Input: part model. Units: mm. Frame: model coordinates. A direction names the side the tool comes from. Round coordinates to 2 decimals unless told otherwise and drop trailing zeros. Loops run counter-clockwise (first coordinate to the right, second up) from the corner with the lowest first, then second, coordinate; pieces in that order, holes last. Notation, with made-up numbers: (-36.75, 69.5) -> (-1.75, 69.5) arc R22 cw to (-1.75, 94.5) -> close; hole circle Ø3 at (78, 26). An arc over 180 degrees is marked (long way). Answer in a Markdown table with one row per item. Add a question column.
Q1. Section A-A, the plane y = -0.5. Output: boundary loops of the cut face in (x, z).
Q2. Mould query, pull axis Z, two halves, no side actions, for faces 1 (the face through (-4.757, 11.598, -0.528)), 2 (the face through (-0.54, -2.44, -0.49)), 3 (the face through (-2, -2, 0)). Classes: pulls with the +Z half, pulls with the -Z half, needs draft (parallel to the pull), parting line crosses it, or undercut.
Q3. Ray query, L1, parallel to Y at x = 8, z = -0.6; L2, parallel to Y at x = 3.75, z = -0.3; L3, parallel to X at y = -6.75, z = -0.1. Return the intervals inside material, ascending. Write a range as from..to.
Q4. Reachability of faces 4 (the face through (4.94, 12.67, -0.49)), 5 (the face through (5.637, 2.848, -0.493)), 6 (the face through (7.3, 0, -0.5)), 7 (the face through (-7.3, 0, -0.5)) from +Z, -Z, +X, -X, +Y, -Y: full face, straight path, thin tool, end or side. Return the list, or none.
Q5. Section B-B, the plane x = -7.75. Give the number of separate pieces and of enclosed holes in the cut face, and give its area (3 significant figures).
Q6. Pin query (flat end, axial travel): pin 1 (0.5 mm diameter, centred on x = 2.5, z = -0.5, fed in from +Y); pin 2 (0.5 mm diameter, centred on y = -7.5, z = -0.5, fed in from -X). Return the tip coordinate at first contact, or that it passes through.
```python
from build123d import *

# Parameters (mm, degrees)
SKETCH1_R           = 2.5
BOSS_EXTRUDE1_DEPTH = 1
BOSS_EXTRUDE2_DEPTH = 1
CUT_EXTRUDE1_START  = -1
SKETCH5_R           = 0.5
CUT_EXTRUDE1_DEPTH  = 20.707970143
CIRPATTERN4_COUNT   = 8


with BuildPart() as part:
    # Sketch1 → Boss-Extrude1 (new body)
    with BuildSketch(Plane.XY):
        Polygon((-6, 0), (-6, 4.000001453), (-8.5, 4.000001453), (-8.5, 6), (-6, 6), (-4.242640687, 4.242640687), (-1.414212535, 7.071068839), (-3.181979488, 8.838835792), (-1.767766953, 10.253048327), (0, 8.485281374), (0, 6), (4.000001453, 6), (4.000001453, 8.5), (6, 8.5), (6, 6), (4.242640687, 4.242640687), (7.071068839, 1.414212535), (8.838835792, 3.181979488), (10.253048327, 1.767766953), (8.485281374, 0), (6, 0), (6, -4.000001453), (8.5, -4.000001453), (8.5, -6), (6, -6), (4.242640687, -4.242640687), (1.414212535, -7.071068839), (3.181979488, -8.838835792), (1.767766953, -10.253048327), (0, -8.485281374), (0, -6), (-4.000001453, -6), (-4.000001453, -8.5), (-6, -8.5), (-6, -6), (-4.242640687, -4.242640687), (-7.071068839, -1.414212535), (-8.838835792, -3.181979488), (-10.253048327, -1.767766953), (-8.485281374, 0), align=None)
        Circle(SKETCH1_R, mode=Mode.SUBTRACT)
    extrude(amount=-BOSS_EXTRUDE1_DEPTH)

    # Sketch2 → Boss-Extrude2 (add)
    with BuildSketch(Plane.XY):
        with BuildLine():
            Line((6, 8.5), (4.000001453, 8.5))
            add(Edge.make_bspline(
                [(4.000001453, 8.5), (4.535044761, 9.851871254), (2.785677296, 10.626331859), (1.69748686, 10.584769031)],
                knots=[0, 0, 0, 0, 1, 1, 1, 1], degree=3))
            ThreePointArc((1.69748686, 10.584769031), (5.000000726, 12.6701636), (8.302514593, 10.584769031))
            add(Edge.make_bspline(
                [(6, 8.5), (5.464956692, 9.851871254), (7.214324157, 10.626331859), (8.302514593, 10.584769031)],
                knots=[0, 0, 0, 0, 1, 1, 1, 1], degree=3))
        make_face()
    boss_extrude2 = extrude(amount=-BOSS_EXTRUDE2_DEPTH)

    # Sketch5 → Cut-Extrude1 (cut)
    with BuildSketch(Plane(origin=(-8.102008287, 0, -8.102008287), x_dir=(0, -1, 0), z_dir=(0.707106781, 0, 0.707106781)).offset(CUT_EXTRUDE1_START)):
        with Locations((-11.065369039, 3.772340366)):
            Circle(SKETCH5_R)
    cut_extrude1 = extrude(amount=CUT_EXTRUDE1_DEPTH, mode=Mode.SUBTRACT)

    # CirPattern4: Boss-Extrude2, Cut-Extrude1 ×8 about axis
    cirpattern4_axis = Axis((0, 0, 0), (0, 0, 1))
    for i in range(1, CIRPATTERN4_COUNT):
        add(boss_extrude2.rotate(cirpattern4_axis, i * 360 / CIRPATTERN4_COUNT))
        add(cut_extrude1.rotate(cirpattern4_axis, i * 360 / CIRPATTERN4_COUNT), mode=Mode.SUBTRACT)


solid = part.part
```
Answer block:
| question | item | result |
|---|---|---|
| 1 | outline | (-8.99, -1) -> (-2.45, -1) -> (-2.45, 0) -> (-8.99, 0) -> close; (2.45, -1) -> (6, -1) -> (6, 0) -> (2.45, 0) -> close |
| 2 | face 1 | undercut |
| 2 | face 2 | needs draft |
| 2 | face 3 | pulls with the +Z half |
| 3 | L1 | -6..-4, 0..2.34, 10.58..11.11 |
| 3 | L2 | -13.45..-11.87, -11.24..-9.46, -4.74..6, 9.81..12.45 |
| 3 | L3 | -6..-4, 0..1.74, 10.2..12.22 |
| 4 | face 4 | +Z, -Z, +Y |
| 4 | face 5 | +Z, -Z |
| 4 | face 6 | +Z, -Z, +X |
| 4 | face 7 | +Z, -Z, -X |
| 5 | separate pieces | 3 |
| 5 | enclosed holes | 0 |
| 5 | area | 4.97 mm^2 |
| 6 | pin 1 | y = 11.9 |
| 6 | pin 2 | x = -6 |
